Geometry: final body of the model. Coordinates: model frame, mm. A direction names the side the tool comes from. Give positions to 0.01 mm unless a question says otherwise; leave off trailing zeros. Write each loop counter-clockwise with the first axis right and the second up, starting at its lowest first coordinate (ties: lowest second). Pieces come first, ordered by that corner, then holes. Notation, with made-up numbers: M 6.5,-7 L 29.5,-7 A30 cw 29.5,32 Z; hole C -19,-0.5 d10. An arc over 180 degrees is marked long. Answer as a JSON object with one key per item and string values.
from build123d import *

# Parameters (mm, degrees)
BOSS_EXTRUDE1_DEPTH = 5
CUT_EXTRUDE1_DEPTH  = 3.5


with BuildPart() as part:
    # Sketch1 → Boss-Extrude1 (new body)
    with BuildSketch(Plane.XY):
        with BuildLine():
            ThreePointArc((83.37845056, 14.469012335), (16.768892688, 70.623970918), (-49.840665185, 14.469012335))
            ThreePointArc((-49.840665185, 14.469012335), (-39.521894243, -0.123659797), (-24.929222112, 10.195111145))
            ThreePointArc((-24.929222112, 10.195111145), (16.768892688, 45.348563357), (58.467007487, 10.195111145))
            ThreePointArc((58.467007487, 10.195111145), (73.059679618, -0.123659797), (83.37845056, 14.469012335))
        make_face()
    extrude(amount=BOSS_EXTRUDE1_DEPTH)

    # Sketch2 → Cut-Extrude1 (cut)
    with BuildSketch(Plane(origin=(0, 0, 0), x_dir=(-1, 0, 0), z_dir=(0, 0, -1))):
        with BuildLine():
            ThreePointArc((46.94943865, 13.837591132), (-16.768892688, 68.310693084), (-80.487224025, 13.837591132))
            ThreePointArc((-80.487224025, 13.837591132), (-72.428258415, 2.767566738), (-61.358234021, 10.826532348))
            ThreePointArc((-61.358234021, 10.826532348), (-16.768892688, 48.946170535), (27.820448646, 10.826532348))
            ThreePointArc((27.820448646, 10.826532348), (38.89047304, 2.767566738), (46.94943865, 13.837591132))
        make_face()
    extrude(amount=-CUT_EXTRUDE1_DEPTH, mode=Mode.SUBTRACT)


solid = part.part
1) Line query: line 1 (X direction, y = 38.5, z = 1.6); line 2 (Y direction, x = -32, z = 2.5); line 3 (Z direction, x = -32.5, y = 22.5). Output: solid intervals per line, ascending. Write a range as from..to.
Geometry check:
{"line 1": "x = -40.76..-37.61, -12.11..-6.31, 39.85..45.65, 71.15..74.3", "line 2": "y = 0.9..4.29, 46.02..49.83", "line 3": "z = 3.5..5"}
2) Cut plane B-B on y = 7.5. Return loops of the section in (x, z), and give its area (3 significant figures).
Geometry check:
{"outline": "M -49.06,0 L -45.78,0 L -45.78,3.5 L -28.99,3.5 L -28.99,0 L -25.71,0 L -25.71,5 L -49.06,5 Z; M 59.25,0 L 62.53,0 L 62.53,3.5 L 79.31,3.5 L 79.31,0 L 82.6,0 L 82.6,5 L 59.25,5 Z", "area": "116 mm2"}
3) Set-up query: faces 4 (the flat face through (16, 51, 5)), 5 (the cylindrical face through (-38.68, 2.737, 1.726)). Return all of +Z, -Z, +X, -X, +Y, -Y with unobstructed straight access to the full face (end or side cutting, diameter ignored); none if empty.
Geometry check:
{"face 4": "+Z, +X, -X, +Y, -Y", "face 5": "-Z"}
4) Pull-direction query (Y, two-part tool) for faces 1 (the cylindrical face through (18.09, 70.61, 2.46)), 2 (the cylindrical face through (17.663, 48.937, 1.726)), 3 (the flat face through (16, 46, 0)); classes: pulls with the +Y half, pulls with the -Y half, needs draft (parallel to the pull), parting line crosses it, or undercut.
Geometry check:
{"face 1": "pulls with the +Y half", "face 2": "undercut", "face 3": "needs draft"}
5) Cut plane D-D on y = 65. Return loops of the section in (x, z).
Geometry check:
{"outline": "M -10.22,0 L -3.63,0 L -3.63,3.5 L 37.17,3.5 L 37.17,0 L 43.76,0 L 43.76,5 L -10.22,5 Z"}
6) Contact query for flat-ended pins moving along their axis: P1, Ø1, axis at y = 17.5, z = 4, coming from the -X side; P2, Ø1.5, axis at y = 52, z = 3, coming from the -X side; P3, Ø2, axis at y = 54, z = 2.5, coming from the +X side. Output: stop coordinate, or through.
Geometry check:
{"P1": "stops at x = -49.36", "P2": "stops at x = -30.6", "P3": "stops at x = 62.28"}
7) Cut plane C-C on x = -41. Return loops of the section in (y, z), and give its area (3 significant figures).
Geometry check:
{"outline": "M 0.22,0 L 3.35,0 L 3.35,3.5 L 32.5,3.5 L 32.5,0 L 38.12,0 L 38.12,5 L 0.22,5 Z", "area": "87.4 mm2"}
